Work out the finished part from the listing and answer in its coordinate system (mm). A direction names the side the tool comes from. Round coordinates to 2 decimals unless told otherwise and drop trailing zeros. Order: outer loops, then holes, each group sorted by start corner. A loop starts at its lowest first (then second) coordinate and runs counter-clockwise, first axis right, second up. Notation, with made-up numbers: (24.5, -2.75) -> (31.5, -2.75) arc R19 ccw to (31.5, 29.25) -> close; hole circle Ø11 at (24.25, 66.25). An arc over 180 degrees is marked (long way). Use one line per item in the form item = value.
```python
from build123d import *

# Parameters (mm, degrees)
SKETCH2_W             = 3
SKETCH2_H             = 20
BOSS_EXTRUDE1_DEPTH   = 8
BOSS_EXTRUDE1_2_DEPTH = 8
SKETCH3_W             = 35
SKETCH3_H             = 20
BOSS_EXTRUDE2_DEPTH   = 8
CUT_EXTRUDE1_DEPTH    = 100
FILLET1_R             = 2


with BuildPart() as part:
    # Sketch2 → Boss-Extrude1 (new body)
    with BuildSketch(Plane.XY):
        with Locations((-5.6, 0)):
            Rectangle(SKETCH2_W, SKETCH2_H)
    extrude(amount=BOSS_EXTRUDE1_DEPTH)



with BuildPart() as body_2:
    # Sketch2 → Boss-Extrude1 2 (new body)
    with BuildSketch(Plane.XY):
        with Locations((5.6, 0)):
            Rectangle(SKETCH2_W, SKETCH2_H)
    extrude(amount=BOSS_EXTRUDE1_2_DEPTH)


with BuildPart() as part_1:
    add(part.part)

    add(body_2.part)  # Boss-Extrude2 merges body 2
    # Sketch3 → Boss-Extrude2 (add)
    with BuildSketch(Plane.XY.offset(8)):
        Rectangle(SKETCH3_W, SKETCH3_H)
    extrude(amount=BOSS_EXTRUDE2_DEPTH)

    # Sketch4 → Cut-Extrude1 (cut)
    with BuildSketch(Plane(origin=(17.5, 0, 0), x_dir=(0, 0, -1), z_dir=(1, 0, 0))):
        with BuildLine():
            Line((-8.650350687, 10), (-18.749318475, 11.146699317))
            Line((-18.749318475, 11.146699317), (-17.556068679, -8.149022999))
            Line((-17.556068679, -8.149022999), (-16, -10))
            add(Edge.make_bspline(
                [(-8.650350687, 10), (-9.760639053, -0.993319635), (-16, -10)],
                knots=[0, 0, 0, 1, 1, 1], degree=2))
        make_face()
    extrude(amount=-CUT_EXTRUDE1_DEPTH, mode=Mode.SUBTRACT)

    # Fillet1
    fillet1_edges = [part_1.edges().sort_by_distance(p)[0] for p in [
        (17.5, 0, 8),
        (-17.5, 0, 8),
        (-7.1, 0, 8),
        (7.1, 0, 8),
    ]]
    fillet(fillet1_edges, radius=FILLET1_R)


solid = part_1.part
```
Item 1: The part is cut by section B-B, the plane z = 7.5. Give the vertices of the cut face in (x, y), and give its area (3 significant figures).
Findings:
outline = (-7.78, -10) -> (-4.1, -10) -> (-4.1, 10) -> (-7.78, 10) -> close; (4.1, -10) -> (7.78, -10) -> (7.78, 10) -> (4.1, 10) -> close
area = 147 mm^2
Item 2: Determine the mould class of faces 4 (the flat face through (-4.1, 0, 4)), 5 (the flat face through (-6, 0, 0)), 6 (the flat face through (-17.5, -7, 12)) for opening direction X: released by +X, released by -X, zero draft, split by the parting line, or undercut.
Findings:
face_4 = undercut
face_5 = zero draft
face_6 = released by -X
Item 3: For faces 1 (the flat face through (0, 0, 8)), 2 (the flat face through (7.1, 0, 3)), 3 (the flat face through (-7.1, 0, 3)), determine the directions among +Z, -Z, +X, -X, +Y, -Y from which every point of the face is accessible in a straight line to the end or side of a thin tool.
Findings:
face_1 = -Z, +Y, -Y
face_2 = -Z, +X, +Y, -Y
face_3 = -Z, -X, +Y, -Y
Item 4: The part is cut by section A-A, the plane z = 1.5. Give the vertices of the cut face in (x, y).
Findings:
outline = (-7.1, -10) -> (-4.1, -10) -> (-4.1, 10) -> (-7.1, 10) -> close; (4.1, -10) -> (7.1, -10) -> (7.1, 10) -> (4.1, 10) -> close
Item 5: Consider line 1 along X through (y, z) = (2, 1.25); line 2 along X through (y, z) = (2.25, 7); line 3 along Z through (x, y) = (-13, -1.5). Determine where each line is inside the solid, lowest interval first.
Findings:
line_1 = -7.1 to -4.1, 4.1 to 7.1
line_2 = -7.37 to -4.1, 4.1 to 7.37
line_3 = 8 to 11.43
Item 6: Flat-ended cylindrical pins translate along their axes: P1, Ø5, axis at x = -10, y = 6, coming from the -Z side; P2, Ø2, axis at x = -8.5, z = 9, coming from the +Y side; P3, Ø4, axis at y = 2, z = 5, coming from the -X side; P4, Ø1.5, axis at x = 12.5, y = -7.5, coming from the +Z side. Find the tip coordinate at first contact, or state that the pin passes through.
Findings:
P1 = 7.2
P2 = 10
P3 = -7.37
P4 = 14.85
